For this review, take the finished solid that the model builds, in its own axes (mm). Face numbers are marked on the shaded views. A direction names the side the tool comes from. Round coordinates to 2 decimals unless told otherwise and drop trailing zeros. Write each loop counter-clockwise with the first axis right and the second up, starting at its lowest first coordinate (ties: lowest second). Pieces come first, ordered by that corner, then holes. Notation, with made-up numbers: M 38,75 L 76,75 A22 ccw 76,82 Z; hole C 32.25,51.5 d2. An arc over 180 degrees is marked long. Use one line per item in the form item = value. Start each with the question number.
Item 1: Draft analysis for pull direction X (two halves, no side actions). For the marked faces 4, 5, 6 and 7, state which applies: released by +X, released by -X, zero draft, split by the parting line, or undercut.
Item 2: Add section C-C (x = 0). State the section outline as (y, z) points.
Item 3: Add section A-A (y = -2.5). State the section outline as (x, z) points.
Item 4: For P1, Ø10, axis at x = 9.5, y = -9.5, coming from the +Z side; P2, Ø9.5, axis at x = 4, z = 6.5, coming from the +Y side; P3, Ø2.5, axis at y = 15, z = 15, coming from the +X side, all flat-tipped, find the tip position at first contact; note any pin that passes through.
Item 5: Add section B-B (z = 36). State the section outline as (x, y) points, and give its area (3 significant figures).
Item 6: Add section D-D (y = 6). State the section outline as (x, z) points, and give its area (3 significant figures).
Item 7: For the marked faces 1, 2 and 3, list the 3-axis set-ups (+Z, -Z, +X, -X, +Y, -Y) from which the entire face can be reached by the end or side of a thin tool; tool diameter is ignored.
Item 8: For line 1 (X direction, y = -14, z = 30.5); line 2 (Y direction, x = 0, z = 2); line 3 (Y direction, x = 0, z = 8.55), list the stretches that pass through material, from the lowest coordinate up. Write a range as [from, to].
from build123d import *

# Parameters (mm, degrees)
SKETCH_1_W                   = 46
SKETCH_1_H                   = 35
EXTRUDE_1_DEPTH              = 39
SKETCH_2_W                   = 30.2
SKETCH_2_H                   = 30
CUT_EXTRUDE_1_DEPTH          = 29
SKETCH_4_W                   = 27.8
SKETCH_4_H                   = 10
CUT_EXTRUDE_2_DEPTH          = 49.541219597
HOLE_WIZARD_M6_2_D           = 6.5
HOLE_WIZARD_M6_2_CBORE_D     = 11
HOLE_WIZARD_M6_2_CBORE_DEPTH = 5
CHAMFER_1_SIZE               = 1.6
FILLET_3_R                   = 10
FILLET_4_R                   = 5


with BuildPart() as part:
    # 草图1 → 凸台-拉伸1 (new body)
    with BuildSketch(Plane.XY):
        Rectangle(SKETCH_1_W, SKETCH_1_H)
    extrude(amount=EXTRUDE_1_DEPTH)

    # 草图2 → 切除-拉伸1 (cut)
    with BuildSketch(Plane.XY.offset(39)):
        with Locations((0, -2.5)):
            Rectangle(SKETCH_2_W, SKETCH_2_H)
    extrude(amount=-CUT_EXTRUDE_1_DEPTH, mode=Mode.SUBTRACT)

    # 草图4 → 切除-拉伸2 (cut, through all)
    with BuildSketch(Plane.XY.offset(39)):
        with Locations((0, 17.5)):
            Rectangle(SKETCH_4_W, SKETCH_4_H)
    extrude(amount=-CUT_EXTRUDE_2_DEPTH, mode=Mode.SUBTRACT)

    # M6 凹头盖螺钉的柱形沉头孔2 (through all)
    with Locations(Plane(origin=(0, 0, 0), x_dir=(-1, 0, 0), z_dir=(0, 0, -1))):
        with Locations((0, -2.5)):
            CounterBoreHole(HOLE_WIZARD_M6_2_D / 2, HOLE_WIZARD_M6_2_CBORE_D / 2, HOLE_WIZARD_M6_2_CBORE_DEPTH)

    # 倒角1
    # the kernel refuses this chamfer: 1.6 mm, written as the material it takes off along each edge
    with BuildSketch(Plane(origin=(13.9, 12.5, 43.114692781), x_dir=(-0.027495876610586285, 0.9996219169112968, 0), z_dir=(0, 0, -1))) as chamfer_1_piece_1_section:
        Polygon((CHAMFER_1_SIZE * 0.999621916911, CHAMFER_1_SIZE * 0.0274958766106), (-CHAMFER_1_SIZE * 0.0274958766106, CHAMFER_1_SIZE * 0.999621916911), (0, 0), align=None)
    chamfer_1_piece_1 = extrude(amount=33.114692781, mode=Mode.PRIVATE)
    chamfer_1_piece_1 = split(chamfer_1_piece_1, bisect_by=Plane(origin=(15.1, 13.06, 24.5), z_dir=(-1, 0, 0)), keep=Keep.TOP, mode=Mode.PRIVATE)
    add(chamfer_1_piece_1, mode=Mode.SUBTRACT)
    with BuildSketch(Plane(origin=(-13.9, 12.5, 43.114692781), x_dir=(0.027495876610586285, 0.9996219169112968, 0), z_dir=(0, 0, -1))) as chamfer_1_piece_2_section:
        Polygon((CHAMFER_1_SIZE * 0.999621916911, -CHAMFER_1_SIZE * 0.0274958766106), (-CHAMFER_1_SIZE * 0.0274958766106, -CHAMFER_1_SIZE * 0.999621916911), (0, 0), align=None)
    chamfer_1_piece_2 = extrude(amount=33.114692781, mode=Mode.PRIVATE)
    chamfer_1_piece_2 = split(chamfer_1_piece_2, bisect_by=Plane(origin=(-15.1, 13.06, 24.5), z_dir=(1, 0, 0)), keep=Keep.TOP, mode=Mode.PRIVATE)
    add(chamfer_1_piece_2, mode=Mode.SUBTRACT)

    # 圆角3
    fillet_3_edges = [part.edges().sort_by_distance(p)[0] for p in [
        (18.45, 17.5, 0),
    ]]
    fillet(fillet_3_edges, radius=FILLET_3_R)

    # 圆角4
    fillet_4_edges = [part.edges().sort_by_distance(p)[0] for p in [
        (23, -5, 0),
        (-23, 17.5, 24.499999812),
        (23, 17.5, 24.5),
        (-23, -5, 0),
        (-23, 14.571067679, 2.928932055),
        (23, 14.571067812, 2.928932188),
    ]]
    fillet(fillet_4_edges, radius=FILLET_4_R)


solid = part.part
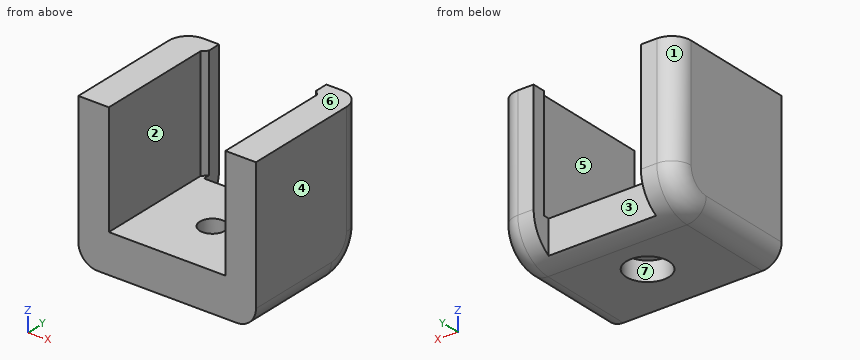
Calculated:
q1.face_4 = released by +X
q1.face_5 = undercut
q1.face_6 = zero draft
q1.face_7 = undercut
q2.outline = M -17.5,0 L -8,0 L -8,5 L -5.75,5 L -5.75,10 L -17.5,10 Z; M 0.75,5 L 3,5 L 3,0 L 7.5,0 A10 ccw 12.5,1.34 L 12.5,10 L 0.75,10 Z
q3.outline = M -23,5 A5 ccw -18,0 L -5.5,0 L -5.5,5 L -3.25,5 L -3.25,10 L -15.1,10 L -15.1,39 L -23,39 Z; M 3.25,5 L 5.5,5 L 5.5,0 L 18,0 A5 ccw 23,5 L 23,39 L 15.1,39 L 15.1,10 L 3.25,10 Z
q4.P1 = 10
q4.P2 = 12.5
q4.P3 = 22.84
q5.outline = M -23,-17.5 L -15.1,-17.5 L -15.1,12.9 L -13.9,14.1 L -13.9,17.5 L -18,17.5 A5 ccw -23,12.5 Z; M 13.9,14.1 L 15.1,12.9 L 15.1,-17.5 L 23,-17.5 L 23,12.5 A5 ccw 18,17.5 L 13.9,17.5 Z
q5.area = 552 mm^2
q6.outline = M -23,5 A5 ccw -18,0 L 18,0 A5 ccw 23,5 L 23,39 L 15.1,39 L 15.1,10 L -15.1,10 L -15.1,39 L -23,39 Z
q6.area = 907 mm^2
q7.face_1 = +Z, -Z, -X, +Y
q7.face_2 = +Z, -Y
q7.face_3 = +Z, -Z, +Y
q8.line_1 = [-23, -15.1], [15.1, 23]
q8.line_2 = [-17.5, -8], [3, 12.5]
q8.line_3 = [-17.5, -5.75], [0.75, 12.5]
